Geometry: final body of the model. Coordinates: model frame, mm. A direction names the side the tool comes from. Give positions to 0.01 mm unless a question says otherwise; leave off trailing zeros. Write each loop counter-clockwise with the first axis right and the second up, starting at its lowest first coordinate (ties: lowest second). Pieces come first, ordered by that corner, then holes.
Q1. Reachability of faces 4 (the flat face through (-16, 12, 1)), 5 (the cylindrical face through (-19.93, -8.66, -4.4)), 6 (the flat face through (18.6, 0, -1)) from +Z, -Z, +X, -X, +Y, -Y: full face, straight path, thin tool, end or side. Return the list, or none.
Q2. Line query: line 1 (X direction, y = 0, z = -2.5); line 2 (X direction, y = -6, z = -3); line 3 (X direction, y = 13.5, z = 0.5). Output: solid intervals per line, ascending.
Q3. Mould query, pull axis X, two halves, no side actions, for faces 1 (the flat face through (-16, -12, 1)), 2 (the flat face through (12, 16, 1)), 3 (the cylindrical face through (22.41, -13.07, -0.6)). Classes: +X half, -X half, draft (parallel to the pull), parting line (faces both ways), or undercut.
Q4. Section B-B (y = 6). Return the cut outline in (x, z), plus the area to 3 significant figures.
Q5. Section C-C (z = -1.25). Return the cut outline in (x, y), plus the area to 3 significant figures.
Q6. Section D-D (x = 3). Return the cut outline in (y, z).
Q7. Pin query (flat end, axial travel): pin 1 Ø1.6 at (y, z) = (16, 1) entering from +X; pin 2 Ø1.6 at (y, z) = (16, 1) entering from -X; pin 3 Ø1.6 at (x, z) = (13, 1) entering from +Y. Return the tip coordinate at first contact, or that it passes through.
Q8. Section A-A (x = 21.5). Return the cut outline in (y, z).
from build123d import *

# Parameters (mm, degrees)
SKETCH016_W     = 41
SKETCH016_H     = 37
SKETCH016_W_2   = 2.7
SKETCH016_H_2   = 10.1
PAD006_DEPTH    = 5
SKETCH017_W     = 1.9
SKETCH017_H     = 10.1
POCKET010_DEPTH = 2.1
PAD008_DEPTH    = 2
PAD007_DEPTH    = 5
FILLET_R        = 2
FILLET004_R     = 2
FILLET005_R     = 2


with BuildPart() as part:
    # Sketch016 → Pad006 (new body)
    with BuildSketch(Plane.XY):
        Rectangle(SKETCH016_W, SKETCH016_H)
        with Locations((-17.25, 0)):
            Rectangle(SKETCH016_W_2, SKETCH016_H_2, mode=Mode.SUBTRACT)
        with Locations((17.25, 0)):
            Rectangle(SKETCH016_W_2, SKETCH016_H_2, mode=Mode.SUBTRACT)
    extrude(amount=-PAD006_DEPTH)

    # Sketch017 (on Face14 of Pad006) → Pocket010 (cut)
    with BuildSketch(Plane(origin=(0, 0, -5), x_dir=(1, 0, 0), z_dir=(0, 0, -1))):
        with Locations((-19.55, 0)):
            Rectangle(SKETCH017_W, SKETCH017_H)
        with Locations((19.55, 0)):
            Rectangle(SKETCH017_W, SKETCH017_H)
    extrude(amount=-POCKET010_DEPTH, mode=Mode.SUBTRACT)

    # Sketch023 (on Face4 of Pocket010) → Pad008 (join)
    with BuildSketch(Plane.XY):
        Polygon((-17, 17), (-12, 17), (-12, 15.5), (-15.5, 15.5), (-15.5, 12), (-17, 12), align=None)
        Polygon((17, 17), (12, 17), (12, 15.5), (15.5, 15.5), (15.5, 12), (17, 12), align=None)
        Polygon((-17, -17), (-12, -17), (-12, -15.5), (-15.5, -15.5), (-15.5, -12), (-17, -12), align=None)
        Polygon((17, -17), (12, -17), (12, -15.5), (15.5, -15.5), (15.5, -12), (17, -12), align=None)
    extrude(amount=PAD008_DEPTH)

    # Sketch018 → Pad007 (join)
    with BuildSketch(Plane.XY):
        Polygon((-23.5, 12.5), (-20.5, 12.5), (-20.5, 18.5), (-28.5, 18.5), (-28.5, -18.5), (-20.5, -18.5), (-20.5, -12.5), (-23.5, -12.5), align=None)
        Polygon((20.5, 12.5), (23.5, 12.5), (23.5, -12.5), (20.5, -12.5), (20.5, -18.5), (28.5, -18.5), (28.5, 18.5), (20.5, 18.5), align=None)
    extrude(amount=-PAD007_DEPTH)

    # Fillet
    fillet_edges = [part.edges().sort_by_distance(p)[0] for p in [
        (-28.5, 18.5, -2.5),
        (-28.5, 0, 0),
        (-28.5, -18.5, -2.5),
        (-28.5, 0, -5),
        (28.5, -18.5, -2.5),
        (28.5, 0, 0),
        (28.5, 18.5, -2.5),
        (28.5, 0, -5),
        (23.5, 0, -5),
        (23.5, 0, 0),
        (-23.5, 0, 0),
        (-23.5, 0, -5),
        (0, -18.5, -5),
        (0, 18.5, -5),
    ]]
    fillet(fillet_edges, radius=FILLET_R)

    # Fillet004
    fillet004_edges = [part.edges().sort_by_distance(p)[0] for p in [
        (-20.5, 8.775, -5),
        (-20.5, -8.775, -5),
        (20.5, 8.775, -5),
        (20.5, -8.775, -5),
    ]]
    fillet(fillet004_edges, radius=FILLET004_R)

    # Fillet005
    fillet005_edges = [part.edges().sort_by_distance(p)[0] for p in [
        (-22, -12.5, -5),
        (-22, 12.5, -5),
        (22, 12.5, -5),
        (-22, 12.5, 0),
        (-22, -12.5, 0),
        (22, 12.5, 0),
        (22, -12.5, 0),
        (22, -12.5, -5),
    ]]
    fillet(fillet005_edges, radius=FILLET005_R)


solid = part.part
Computed:
1. face 4: +Z, +X, -X
1. face 5: -Z
1. face 6: +Z, -Z
2. line 1: x = -28.5 to -23.5, -20.5 to -18.6, -15.9 to 15.9, 18.6 to 20.5, 23.5 to 28.5
2. line 2: x = -28.5 to -23.5, -20.5 to 20.5, 23.5 to 28.5
2. line 3: x = -17 to -15.5, 15.5 to 17
3. face 1: draft
3. face 2: undercut
3. face 3: undercut
4. outline: (-28.5, -3) arc R2 ccw to (-26.5, -5) - (-25.5, -5) arc R2 ccw to (-23.5, -3) - (-23.5, -2) arc R2 ccw to (-25.5, 0) - (-26.5, 0) arc R2 ccw to (-28.5, -2) - close; (-20.5, -3) arc R2 ccw to (-18.5, -5) - (18.5, -5) arc R2 ccw to (20.5, -3) - (20.5, 0) - (-20.5, 0) - close; (23.5, -3) arc R2 ccw to (25.5, -5) - (26.5, -5) arc R2 ccw to (28.5, -3) - (28.5, -2) arc R2 ccw to (26.5, 0) - (25.5, 0) arc R2 ccw to (23.5, -2) - close
4. area: 246 mm2
5. outline: (-28.35, -17.25) arc R2 ccw to (-26.5, -18.5) - (26.5, -18.5) arc R2 ccw to (28.35, -17.25) - (28.35, 17.25) arc R2 ccw to (26.5, 18.5) - (-26.5, 18.5) arc R2 ccw to (-28.35, 17.25) - close; hole (-23.65, -12.65) - (-20.5, -12.65) - (-20.5, 12.65) - (-23.65, 12.65) - close; hole (-18.6, -5.05) - (-15.9, -5.05) - (-15.9, 5.05) - (-18.6, 5.05) - close; hole (15.9, -5.05) - (18.6, -5.05) - (18.6, 5.05) - (15.9, 5.05) - close; hole (20.5, -12.65) - (23.65, -12.65) - (23.65, 12.65) - (20.5, 12.65) - close
5. area: 1,880 mm2
6. outline: (-18.5, -3) arc R2 ccw to (-16.5, -5) - (16.5, -5) arc R2 ccw to (18.5, -3) - (18.5, 0) - (-18.5, 0) - close
7. pin 1: stops at x = 17
7. pin 2: stops at x = -17
7. pin 3: stops at y = 17
8. outline: (-18.5, -3) arc R2 ccw to (-16.5, -5) - (-14.5, -5) arc R2 ccw to (-12.5, -3) - (-12.5, -2) arc R2 ccw to (-14.5, 0) - (-18.5, 0) - close; (12.5, -3) arc R2 ccw to (14.5, -5) - (16.5, -5) arc R2 ccw to (18.5, -3) - (18.5, 0) - (14.5, 0) arc R2 ccw to (12.5, -2) - close
